Design review of the part built by this model. Coordinates are the model's own, in mm. A direction names the side the tool comes from. Round coordinates to 2 decimals unless told otherwise and drop trailing zeros. Write each loop counter-clockwise with the first axis right and the second up, starting at its lowest first coordinate (ties: lowest second). Pieces come first, ordered by that corner, then holes. Notation, with made-up numbers: (39.25, 39) -> (68.25, 39) arc R13 ccw to (68.25, 50) -> close; hole circle Ø4 at (26.25, 17.25). An arc over 180 degrees is marked (long way). Write item = value, one per line. Start each with the question number.
Item 1: Mouldability with a two-part tool opening along Z and no side actions: class faces 4 (the flat face through (-1, 0, 0)), 5 (the flat face through (57, -38, -25.4)), 6 (the flat face through (1, -19, 12.693)), 7 (the flat face through (44.4, -38.6, -19.1)) as released by +Z, released by -Z, zero draft, split by the parting line, or undercut.
Item 2: To check wall thickness, follow L1, parallel to Y at x = -8, z = 2; L2, parallel to Y at x = 2, z = 14; L3, parallel to Z at x = 35, y = -23. State the ranges of each line that lie inside material, in increasing order.
Item 3: Add section A-A, the plane z = -22. State the section outline as (x, y) points.
Item 4: Add section B-B, the plane x = -47. State the section outline as (y, z) points.
Item 5: Machinability: for faces 1 (the flat face through (-44.5, -38.6, -19)), 2 (the flat face through (1, -38, 0)), 3 (the flat face through (1, -25.4, 19)), which of the approach directions +Z, -Z, +X, -X, +Y, -Y give a long, thin tool a straight path to every point of the face, cutting with its end or side? Answer none if there is none.
Item 6: For pin 1 Ø6 at (x, y) = (-25.5, -34) entering from +Z; pin 2 Ø2 at (y, z) = (-27.5, 11) entering from -X; pin 3 Ø6.5 at (x, y) = (6.5, -18) entering from -Z, all flat-tipped, find the tip position at first contact; note any pin that passes through.
Item 7: Add section C-C, the plane y = -19. State the section outline as (x, z) points, then the cut area to 3 significant figures.
Item 8: Add section D-D, the plane y = -11. State the section outline as (x, z) points.
from build123d import *

# Parameters (mm, degrees)
F0_W     = 152.4
F0_H     = 50.8
F1_DEPTH = 76.2
F3_DEPTH = 152.401
F5_DEPTH = 76.201


with BuildPart() as f1:
    # F0 (on Front) → F1 (new body)
    with BuildSketch(Plane.XZ):
        Rectangle(F0_W, F0_H)
    extrude(amount=F1_DEPTH)

    # F2 (on face) → F3 (cut, through all)
    with BuildSketch(Plane.YZ.offset(76.2)):
        Polygon((-25.4, 12.693209), (-25.4, 25.4), (-50.8, 25.4), (-50.8, 12.693209), (-63.5, 12.693209), (-63.5, 0), (-12.7, 0), (-12.7, 12.693209), align=None)
    extrude(amount=-F3_DEPTH, mode=Mode.SUBTRACT)

    # F4 (on face) → F5 (cut, through all)
    with BuildSketch(Plane.XZ.offset(76.2)):
        Polygon((50.8, -12.7), (0, -12.7), (-50.8, -12.7), (-38.1, -25.4), (38.1, -25.4), align=None)
    extrude(amount=-F5_DEPTH, mode=Mode.SUBTRACT)


solid = f1.part
Result set:
q1.face_4 = zero draft
q1.face_5 = released by -Z
q1.face_6 = undercut
q1.face_7 = undercut
q2.L1 = -76.2 to -63.5, -12.7 to 0
q2.L2 = -76.2 to -50.8, -25.4 to 0
q2.L3 = -12.7 to 0, 12.69 to 25.4
q3.outline = (-76.2, -76.2) -> (-41.5, -76.2) -> (-41.5, 0) -> (-76.2, 0) -> close; (41.5, -76.2) -> (76.2, -76.2) -> (76.2, 0) -> (41.5, 0) -> close
q4.outline = (-76.2, -25.4) -> (0, -25.4) -> (0, -16.5) -> (-76.2, -16.5) -> close; (-76.2, -12.7) -> (0, -12.7) -> (0, 25.4) -> (-25.4, 25.4) -> (-25.4, 12.69) -> (-12.7, 12.69) -> (-12.7, 0) -> (-63.5, 0) -> (-63.5, 12.69) -> (-50.8, 12.69) -> (-50.8, 25.4) -> (-76.2, 25.4) -> close
q5.face_1 = +Y, -Y
q5.face_2 = +X, -X
q5.face_3 = +Z, +X, -X
q6.pin_1 = 0
q6.pin_2 = through
q6.pin_3 = -12.7
q7.outline = (-76.2, -25.4) -> (-38.1, -25.4) -> (-50.8, -12.7) -> (50.8, -12.7) -> (38.1, -25.4) -> (76.2, -25.4) -> (76.2, 0) -> (-76.2, 0) -> close; (-76.2, 12.69) -> (76.2, 12.69) -> (76.2, 25.4) -> (-76.2, 25.4) -> close
q7.area = 4,680 mm²
q8.outline = (-76.2, -25.4) -> (-38.1, -25.4) -> (-50.8, -12.7) -> (50.8, -12.7) -> (38.1, -25.4) -> (76.2, -25.4) -> (76.2, 25.4) -> (-76.2, 25.4) -> close
